Source: CAD feature listing. Evaluate the final solid. Frame: model axes, mm. A direction names the side the tool comes from. Coordinates: 2 decimals unless noted, no trailing zeros. Order: outer loops, then holes, each group sorted by start corner. A loop starts at its lowest first (then second) coordinate and runs counter-clockwise, first axis right, second up. Notation, with made-up numbers: (30, 37.5) - (63, 37.5) arc R18 cw to (63, 68.5) - close; hole circle Ø10 at (-12, 37). An arc over 180 degrees is marked (long way). One line per question, with ' | ' between items.
from build123d import *

# Parameters (mm, degrees)
SKETCH1_R           = 12.5
BOSS_EXTRUDE1_DEPTH = 25
SKETCH2_R           = 11
BOSS_EXTRUDE2_DEPTH = 2
BOSS_EXTRUDE3_START = 30
SKETCH3_R           = 12.5
BOSS_EXTRUDE3_DEPTH = 30
SKETCH4_R           = 4.5
BOSS_EXTRUDE4_DEPTH = 2
FILLET1_R           = 2
FILLET2_R           = 1
FILLET3_R           = 1
SKETCH5_R           = 2
BOSS_EXTRUDE5_DEPTH = 12
CUT_EXTRUDE1_START  = -9
CUT_EXTRUDE1_DEPTH  = 9


with BuildPart() as part:
    # Sketch1 → Boss-Extrude1 (new body)
    with BuildSketch(Plane(origin=(0, 0, 0), x_dir=(1, 0, 0), z_dir=(0, 1, 0))):
        with Locations(Location((0, 0, 0), (0, 0, 270))):
            Circle(SKETCH1_R)
    extrude(amount=BOSS_EXTRUDE1_DEPTH)

    # Sketch2 → Boss-Extrude2 (add)
    with BuildSketch(Plane.XZ):
        with Locations(Location((0, 0, 0), (0, 0, 270))):
            Circle(SKETCH2_R)
    extrude(amount=BOSS_EXTRUDE2_DEPTH)

    # Sketch3 → Boss-Extrude3 (add)
    with BuildSketch(Plane.XZ.offset(2).offset(BOSS_EXTRUDE3_START)):
        with Locations(Location((0, 0, 0), (0, 0, 90))):
            Circle(SKETCH3_R)
    extrude(amount=-BOSS_EXTRUDE3_DEPTH)

    # Sketch4 → Boss-Extrude4 (add)
    with BuildSketch(Plane.XZ.offset(-25)):
        with Locations(Location((0, -2.5, 0), (0, 0, 270))):
            Circle(SKETCH4_R)
    extrude(amount=-BOSS_EXTRUDE4_DEPTH)

    # Fillet1
    fillet1_edges = [part.edges().sort_by_distance(p)[0] for p in [
        (0, 25, -12.5),
    ]]
    fillet(fillet1_edges, radius=FILLET1_R)

    # Fillet2
    fillet2_edges = [part.edges().sort_by_distance(p)[0] for p in [
        (0, -2, -12.5),
    ]]
    fillet(fillet2_edges, radius=FILLET2_R)

    # Fillet3
    fillet3_edges = [part.edges().sort_by_distance(p)[0] for p in [
        (0, 27, 2),
    ]]
    fillet(fillet3_edges, radius=FILLET3_R)

    # Sketch5 → Boss-Extrude5 (add)
    with BuildSketch(Plane(origin=(0, 27, 0), x_dir=(1, 0, 0), z_dir=(0, 1, 0))):
        with Locations(Location((0, 2.5, 0), (0, 0, 90))):
            Circle(SKETCH5_R)
    extrude(amount=BOSS_EXTRUDE5_DEPTH)

    # Sketch10 → Cut-Extrude1 (cut)
    with BuildSketch(Plane(origin=(0, 39, 0), x_dir=(1, 0, 0), z_dir=(0, 1, 0)).offset(CUT_EXTRUDE1_START)):
        with BuildLine():
            Line((-0.731515286, 4.361420261), (-1.103703337, 0.832115428))
            ThreePointArc((-1.103703337, 0.832115428), (-1.988970839, 2.709749856), (-0.731515286, 4.361420261))
        make_face()
    extrude(amount=CUT_EXTRUDE1_DEPTH, mode=Mode.SUBTRACT)


solid = part.part
(1) Cut plane B-B (y = -1). Return the cut outline in (x, z), and give its area (3 significant figures).
Taken from the geometry:
outline: circle Ø22 at (0, 0) | area: 380 mm²
(2) Material intervals for L1, parallel to X at y = -3.5, z = 0.25; L2, parallel to Y at x = 7, z = -2.5; L3, parallel to Y at x = 6.5, z = 9, sorted ascending. Write a range as from..to.
Taken from the geometry:
L1: x = -12.5..12.5 | L2: y = -32..25 | L3: y = -32..-2, 0..24.91
(3) Set-up query: faces 5 (the flat face through (-0.915, 34.437, -2.621)), 6 (the cylindrical face through (1.774, 32.916, -3.423)), 7 (the cylindrical face through (3.755, 11.339, 11.923)). Return all of +Z, -Z, +X, -X, +Y, -Y with unobstructed straight access to the full face (end or side cutting, diameter ignored); none if empty.
Taken from the geometry:
face 5: -Z, -X, +Y | face 6: +Y | face 7: +Y, -Y
(4) Cut plane C-C (y = 9). Return the cut outline in (x, z), and give its area (3 significant figures).
Taken from the geometry:
outline: circle Ø25 at (0, 0) | area: 491 mm²
(5) Pull-direction query (Y, two-part tool) for faces 1 (the flat face through (-10, 0, 5)), 2 (the flat face through (-1.4, 30, -2.6)), 3 (the cylindrical face through (-10.74, -0.99, 2.38)), 4 (the cylindrical face through (3.04, 25.49, 0.82)); classes: pulls with the +Y half, pulls with the -Y half, needs draft (parallel to the pull), parting line crosses it, or undercut.
Taken from the geometry:
face 1: undercut | face 2: pulls with the +Y half | face 3: undercut | face 4: needs draft
(6) Pin query (flat end, axial travel): P1, Ø7.5, axis at x = -1.5, z = -1.5, coming from the +Y side; P2, Ø1, axis at y = 18.5, z = -10, coming from the -X side; P3, Ø4, axis at x = -5, y = 4, coming from the -Z side; P4, Ø1.5, axis at x = -4.5, y = 24, coming from the -Z side. Return the tip coordinate at first contact, or that it passes through.
Taken from the geometry:
P1: stops at y = 39 | P2: stops at x = -8.12 | P3: stops at z = -12.13 | P4: stops at z = -11.8
(7) Cut plane A-A (x = 0). Return the cut outline in (y, z), and give its area (3 significant figures).
Taken from the geometry:
outline: (-32, -12.5) - (-3, -12.5) arc R1 ccw to (-2, -11.5) - (-2, -11) - (0, -11) - (0, -12.5) - (23, -12.5) arc R2 ccw to (25, -10.5) - (25, -7) - (26, -7) arc R1 ccw to (27, -6) - (27, -4.5) - (39, -4.5) - (39, -0.5) - (27, -0.5) - (27, 1) arc R1 ccw to (26, 2) - (25, 2) - (25, 10.5) arc R2 ccw to (23, 12.5) - (0, 12.5) - (0, 11) - (-2, 11) - (-2, 11.5) arc R1 ccw to (-3, 12.5) - (-32, 12.5) - close | area: 1,480 mm²
